For this review, use the dimensioned drawing (mm, ordinates from the lowest corner) and the shaded views. Coordinates: 2 decimals unless noted, no trailing zeros. Loops run counter-clockwise (first coordinate to the right, second up) from the corner with the lowest first, then second, coordinate; pieces in that order, holes last.
1. To check wall thickness, follow probe 1 along X at (y, z) = (11.5, 36.5); probe 2 along Y at (x, z) = (51.5, 506.5). State the ranges of each line that lie inside material, in increasing order.
2. Take a section at B-B, the plane z = 465.5. State the section outline as (x, y) points, then the cut area to 3 significant figures.
3. Take a section at A-A, the plane y = 15.25. State the section outline as (x, z) points.
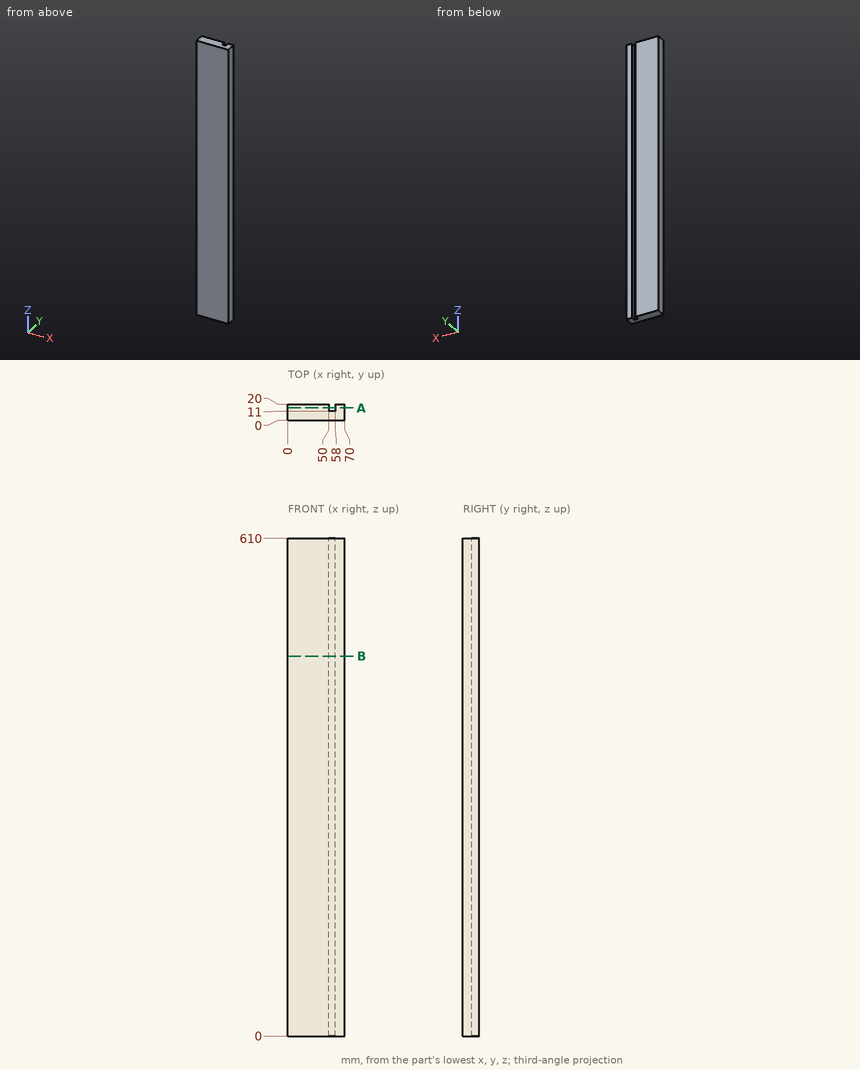
Results list:
1. probe 1: x = 0 to 50, 58 to 70
1. probe 2: y = 0 to 11
2. outline: (0, 0) - (70, 0) - (70, 20) - (58, 20) - (58, 11) - (50, 11) - (50, 20) - (0, 20) - close
2. area: 1,330 mm2
3. outline: (0, 0) - (50, 0) - (50, 610) - (0, 610) - close; (58, 0) - (70, 0) - (70, 610) - (58, 610) - close
